Geometry check sheet. Reference: the model listing, model coordinates, mm. Face numbers are marked on the shaded views. A direction names the side the tool comes from. Give positions to 0.01 mm unless a question says otherwise; leave off trailing zeros. Loops run counter-clockwise (first coordinate to the right, second up) from the corner with the lowest first, then second, coordinate; pieces in that order, holes last.
```python
from build123d import *

# Parameters (mm, degrees)
F0_R     = 10
F1_DEPTH = 5
F2_R     = 10
F3_DEPTH = 12.5


with BuildPart() as f1:
    # F0 (on Top) → F1 (new body, symmetric)
    with BuildSketch(Plane.XY):
        with BuildLine():
            Line((-20, -20), (0, -20))
            ThreePointArc((0, -20), (20, 0), (0, 20))
            Line((0, 20), (-20, 20))
            Line((-20, 20), (-20, -20))
        make_face()
        Circle(F0_R, mode=Mode.SUBTRACT)
    extrude(amount=F1_DEPTH, both=True)

    # F2 (on Front) → F3 (join, symmetric)
    with BuildSketch(Plane.XZ):
        with BuildLine():
            ThreePointArc((-10, 5), (-17.071068, 7.928932), (-20, 15))
            Line((-20, 15), (-20, 25))
            Line((-20, 25), (-50, 25))
            ThreePointArc((-50, 25), (-57.071068, 22.071068), (-60, 15))
            Line((-60, 15), (-60, -15))
            ThreePointArc((-60, -15), (-57.071068, -22.071068), (-50, -25))
            Line((-50, -25), (-20, -25))
            Line((-20, -25), (-20, -15))
            ThreePointArc((-20, -15), (-17.071068, -7.928932), (-10, -5))
            Line((-10, -5), (-20, -5))
            Line((-20, -5), (-20, 5))
            Line((-20, 5), (-10, 5))
        make_face()
        with Locations((-40, 5)):
            Circle(F2_R, mode=Mode.SUBTRACT)
    extrude(amount=F3_DEPTH, both=True)


solid = f1.part
```
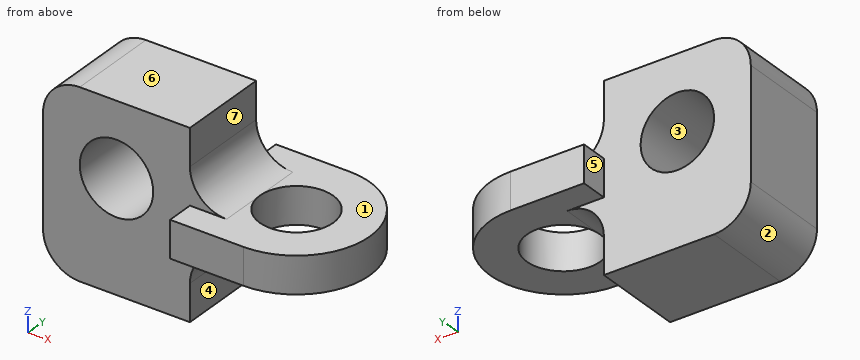
1) Sectioned sample at A-A on z = -3. Enter the section's corners in (x, y), plus the area to 3 significant figures.
2) Sectioned sample at C-C on y = -5. Enter the section's corners in (x, z).
3) Sectioned sample at D-D on y = 11. Enter the section's corners in (x, z), plus the area to 3 significant figures.
4) Sectioned sample at B-B on x = -40. Enter the section's corners in (y, z), plus the area to 3 significant figures.
5) Mould release check, pull along Z, two halves, no side actions. Record for the marked faces 1, 2 and 3: +Z half, -Z half, draft (parallel to the pull), parting line (faces both ways), or undercut.
6) Scan lines: line 1 along Z through (x, y) = (-40, 0); line 2 along Z through (x, y) = (-7, 12); line 3 along Z through (x, y) = (-32, -10). Record each from-to range of solid material in increasing order.
7) Depth check by flat-ended pin: P1, Ø12, axis at y = -8.5, z = 1, coming from the +X side; P2, Ø6, axis at y = 16, z = 0.5, coming from the -X side; P3, Ø11, axis at y = 0, z = 21.5, coming from the +X side; P4, Ø16, axis at x = 0, y = 0, coming from the -Z side. Enter the tip coordinate at first touch or a pass-through.
8) Tool access check on the marked faces 4, 5, 6 and 7. Record the directions out of +Z, -Z, +X, -X, +Y, -Y that give a thin tool (end or side, any length) a straight path to the whole face; none if there is none.
Determined:
1. outline: (-60, -12.5) - (-46, -12.5) - (-46, 12.5) - (-60, 12.5) - close; (-34, -12.5) - (-20, -12.5) - (-20, -20) - (0, -20) arc R20 ccw to (0, 20) - (-20, 20) - (-20, 12.5) - (-34, 12.5) - close; hole circle Ø20 at (0, 0)
1. area: 1,810 mm2
2. outline: (-60, -15) arc R10 ccw to (-50, -25) - (-20, -25) - (-20, -15) arc R10 cw to (-10, -5) - (-8.66, -5) - (-8.66, 5) - (-10, 5) arc R10 cw to (-20, 15) - (-20, 25) - (-50, 25) arc R10 ccw to (-60, 15) - close; (8.66, -5) - (19.36, -5) - (19.36, 5) - (8.66, 5) - close; hole circle Ø20 at (-40, 5)
3. outline: (-60, -15) arc R10 ccw to (-50, -25) - (-20, -25) - (-20, -15) arc R10 cw to (-10, -5) - (16.7, -5) - (16.7, 5) - (-10, 5) arc R10 cw to (-20, 15) - (-20, 25) - (-50, 25) arc R10 ccw to (-60, 15) - close; hole circle Ø20 at (-40, 5)
3. area: 2,050 mm2
4. outline: (-12.5, -25) - (12.5, -25) - (12.5, -5) - (-12.5, -5) - close; (-12.5, 15) - (12.5, 15) - (12.5, 25) - (-12.5, 25) - close
4. area: 750 mm2
5. face 1: +Z half
5. face 2: -Z half
5. face 3: undercut
6. line 1: z = -25 to -5, 15 to 25
6. line 2: z = -5 to 5
6. line 3: z = -25 to -1, 11 to 25
7. P1: stops at x = 19.84
7. P2: stops at x = -20
7. P3: stops at x = -20
7. P4: passes through
8. face 4: -Z, +X, +Y, -Y
8. face 5: +Z, -Z, -X, +Y
8. face 6: +Z, +X, -X, +Y, -Y
8. face 7: +Z, +X, +Y, -Y
